Build history of the part. All positions in model axes, mm. Give positions to 0.01 mm unless a question says otherwise; leave off trailing zeros. Loops run counter-clockwise (first coordinate to the right, second up) from the corner with the lowest first, then second, coordinate; pieces in that order, holes last.
1) Band-saw the part on A-A on z = -2.5. List the corners of the cut face in (x, y), then the cut area to 3 significant figures.
2) Wall check: line 1 (Y direction, x = -7.25, z = 2.75); line 2 (X direction, y = 0.5, z = 9.5); line 3 (Z direction, x = -10.25, y = 1.05). Give the ranges that are in metal, low to high.
3) Band-saw the part on C-C on y = -0.9. List the corners of the cut face in (x, z), then the cut area to 3 significant figures.
4) Band-saw the part on D-D on z = 6.25. List the corners of the cut face in (x, y).
5) Band-saw the part on B-B on x = 0. List the corners of the cut face in (y, z).
6) Flat gauge pin, fed straight in: P1, Ø4, axis at x = -2, z = -7, coming from the -Y side. Where does the tip first touch, or does it go through?
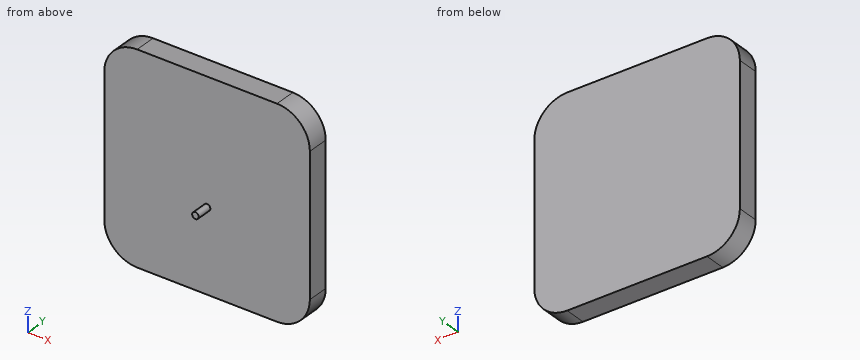
```python
from build123d import *

# Parameters (mm, degrees)
SKETCH1_W           = 25
SKETCH1_H           = 25
BOSS_EXTRUDE1_DEPTH = 2.6
FILLET1_R           = 4
SKETCH2_R           = 0.4
BOSS_EXTRUDE2_DEPTH = 1.9


with BuildPart() as part:
    # Sketch1 → Boss-Extrude1 (new body)
    with BuildSketch(Plane(origin=(0, 0, 0), x_dir=(1, 0, 0), z_dir=(0, 1, 0))):
        Rectangle(SKETCH1_W, SKETCH1_H)
    extrude(amount=BOSS_EXTRUDE1_DEPTH)

    # Fillet1
    fillet1_edges = [part.edges().sort_by_distance(p)[0] for p in [
        (12.5, 1.3, 12.5),
        (-12.5, 1.3, 12.5),
        (-12.5, 1.3, -12.5),
        (12.5, 1.3, -12.5),
    ]]
    fillet(fillet1_edges, radius=FILLET1_R)

    # Sketch2 → Boss-Extrude2 (add)
    with BuildSketch(Plane.XZ):
        with Locations(Location((0, -2.5, 0), (0, 0, 270))):  # turned: the seam where the file's is
            Circle(SKETCH2_R)
    extrude(amount=BOSS_EXTRUDE2_DEPTH)


solid = part.part
```
Findings below:
1. outline: (-12.5, 0) - (-0.4, 0) - (-0.4, -1.9) - (0.4, -1.9) - (0.4, 0) - (12.5, 0) - (12.5, 2.6) - (-12.5, 2.6) - close
1. area: 66.5 mm2
2. line 1: y = 0 to 2.6
2. line 2: x = -12.37 to 12.37
2. line 3: z = -12.1 to 12.1
3. outline: circle Ø0.8 at (0, -2.5)
3. area: 0.503 mm2
4. outline: (-12.5, 0) - (12.5, 0) - (12.5, 2.6) - (-12.5, 2.6) - close
5. outline: (-1.9, -2.9) - (0, -2.9) - (0, -12.5) - (2.6, -12.5) - (2.6, 12.5) - (0, 12.5) - (0, -2.1) - (-1.9, -2.1) - close
6. P1: stops at y = 0
